Design review of the part built by this model. Coordinates are the model's own, in mm. A direction names the side the tool comes from. Round coordinates to 2 decimals unless told otherwise and drop trailing zeros. Order: outer loops, then holes, each group sorted by start corner. A loop starts at its lowest first (then second) coordinate and runs counter-clockwise, first axis right, second up. Notation, with made-up numbers: (12.25, -4.75) - (20.25, -4.75) arc R30 ccw to (20.25, 33.25) - close; hole circle Ø5 at (21.25, 12). An arc over 180 degrees is marked (long way). Use CSV: the item, a comma, the result in double quotes. Start each with the question number.
from build123d import *

# Parameters (mm, degrees)
F1_DEPTH = 5
F2_R     = 18.5
F3_DEPTH = 9
F4_R     = 16.5
F5_DEPTH = 25
F6_R     = 81
F7_DEPTH = 2.84
F8_R     = 17.4877623158
F9_DEPTH = 25


with BuildPart() as f1:
    # F0 (on Top) → F1 (new body)
    with BuildSketch(Plane.XY):
        with BuildLine():
            Line((18.5, 0), (18.5, 10.68097998))
            Line((18.5, 10.68097998), (9.2500001737, 16.0214698697))
            ThreePointArc((9.2500001737, 16.0214698697), (16.0214700202, 9.2499999131), (18.5, 0))
        make_face()
        with BuildLine():
            ThreePointArc((9.2500002367, -16.0214698334), (16.0214700383, -9.2499998817), (18.5, 0))
            ThreePointArc((18.5, 0), (16.0214700202, 9.2499999131), (9.2500001737, 16.0214698697))
            ThreePointArc((9.2500001737, 16.0214698697), (3.666e-07, 18.5), (-9.2499995387, 16.0214702364))
            ThreePointArc((-9.2499995387, 16.0214702364), (-16.0214698368, 9.2500002307), (-18.5, 0))
            ThreePointArc((-18.5, 0), (-16.0214699908, -9.2499999641), (-9.2500000719, -16.0214699285))
            ThreePointArc((-9.2500000719, -16.0214699285), (9.51e-08, -18.5), (9.2500002367, -16.0214698334))
        make_face()
        with BuildLine():
            Line((18.5, -10.68097998), (18.5, 0))
            ThreePointArc((18.5, 0), (16.0214700383, -9.2499998817), (9.2500002367, -16.0214698334))
            Line((9.2500002367, -16.0214698334), (18.5, -10.68097998))
        make_face()
        with BuildLine():
            ThreePointArc((-9.2499995387, 16.0214702364), (3.666e-07, 18.5), (9.2500001737, 16.0214698697))
            Line((9.2500001737, 16.0214698697), (0, 21.36195996))
            Line((0, 21.36195996), (-9.2499995387, 16.0214702364))
        make_face()
        with BuildLine():
            Line((0, -21.36195996), (9.2500002367, -16.0214698334))
            ThreePointArc((9.2500002367, -16.0214698334), (9.51e-08, -18.5), (-9.2500000719, -16.0214699285))
            Line((-9.2500000719, -16.0214699285), (0, -21.36195996))
        make_face()
        with BuildLine():
            ThreePointArc((-18.5, 0), (-16.0214698368, 9.2500002307), (-9.2499995387, 16.0214702364))
            Line((-9.2499995387, 16.0214702364), (-18.5, 10.68097998))
            Line((-18.5, 10.68097998), (-18.5, 0))
        make_face()
        with BuildLine():
            Line((-18.5, -10.68097998), (-9.2500000719, -16.0214699285))
            ThreePointArc((-9.2500000719, -16.0214699285), (-16.0214699908, -9.2499999641), (-18.5, 0))
            Line((-18.5, 0), (-18.5, -10.68097998))
        make_face()
    extrude(amount=F1_DEPTH)

    # F2 (on face) → F3 (join)
    with BuildSketch(Plane.XY.offset(5)):
        Circle(F2_R)
    extrude(amount=F3_DEPTH)

    # F4 (on face) → F5 (cut)
    with BuildSketch(Plane.XY.offset(14)):
        Circle(F4_R)
    extrude(amount=-F5_DEPTH, mode=Mode.SUBTRACT)

    # F6 (on Top) → F7 (join)
    with BuildSketch(Plane.XY):
        Circle(F6_R)
    extrude(amount=-F7_DEPTH)

    # F8 (on face) → F9 (cut)
    with BuildSketch(Plane.XY):
        Circle(F8_R)
    extrude(amount=-F9_DEPTH, mode=Mode.SUBTRACT)


solid = f1.part
Q1. Tool access review of faces 4 (the flat face through (17, 9, 5)), 5 (the flat face through (18.5, 0, 2)), 6 (the flat face through (17, -10, 5)), 7 (the flat face through (6.4, -15.5, 0)), 8 (the flat face through (-17, -10, 5)): name each direction out of +Z, -Z, +X, -X, +Y, -Y from which nothing blocks a thin tool from reaching the whole face with its end or side.
Q2. Clearance check with flat-ended pins moving along their axes: pin 1 (2 mm diameter, centred on x = 27, y = -49, fed in from +Z); pin 2 (4 mm diameter, centred on y = -2.5, z = 2.5, fed in from +X); pin 3 (5 mm diameter, centred on y = 58.5, z = -1, fed in from +X). State where each tip first meets the part, or that it passes through.
Q3. The part is to be moulded in two halves that separate along X. For faces 1 (the flat face through (-18.5, 0, 2)), 2 (the flat face through (-17, 9, 5)), 3 (the cylindrical face through (15.24, -6.32, 7.1)), say which applies: +X half, -X half, draft (parallel to the pull), parting line (faces both ways), or undercut.
Q4. Take a section at B-B (z = 12). State the section outline as (x, y) points, plus the area to 3 significant figures.
Q5. Take a section at D-D (x = 57.5). State the section outline as (y, z) points, plus the area to 3 significant figures.
Q6. Take a section at C-C (x = -4). State the section outline as (y, z) points.
Q7. Take a section at A-A (y = -5.5). State the section outline as (x, z) points.
Q8. For L1, parallel to Y at x = 0, z = 6.75; L2, parallel to X at y = 1, z = 7.5; L3, parallel to Y at x = 0, z = -1.4, list the stretches that pass through material, from the lowest coordinate up. Write a range as [from, to].
Findings below:
1,face 4,"+Z, +X, +Y"
1,face 5,"+Z, +X, +Y, -Y"
1,face 6,"+Z, +X, -Y"
1,face 7,"-Z"
1,face 8,"+Z, -X, -Y"
2,pin 1,"stops at z = 0"
2,pin 2,"stops at x = 18.5"
2,pin 3,"stops at x = 58.52"
3,face 1,"-X half"
3,face 2,"draft"
3,face 3,"undercut"
4,outline,"circle Ø37 at (0, 0); hole circle Ø33 at (0, 0)"
4,area,"220 mm^2"
5,outline,"(-57.05, -2.84) - (57.05, -2.84) - (57.05, 0) - (-57.05, 0) - close"
5,area,"324 mm^2"
6,outline,"(-80.9, -2.84) - (-17.02, -2.84) - (-17.02, 0) - (-16.01, 0) - (-16.01, 14) - (-18.06, 14) - (-18.06, 5) - (-19.05, 5) - (-19.05, 0) - (-80.9, 0) - close; (16.01, 0) - (17.02, 0) - (17.02, -2.84) - (80.9, -2.84) - (80.9, 0) - (19.05, 0) - (19.05, 5) - (18.06, 5) - (18.06, 14) - (16.01, 14) - close"
7,outline,"(-80.81, -2.84) - (-16.6, -2.84) - (-16.6, 0) - (-15.56, 0) - (-15.56, 14) - (-17.66, 14) - (-17.66, 5) - (-18.5, 5) - (-18.5, 0) - (-80.81, 0) - close; (15.56, 0) - (16.6, 0) - (16.6, -2.84) - (80.81, -2.84) - (80.81, 0) - (18.5, 0) - (18.5, 5) - (17.66, 5) - (17.66, 14) - (15.56, 14) - close"
8,L1,"y = [-18.5, -16.5], [16.5, 18.5]"
8,L2,"x = [-18.47, -16.47], [16.47, 18.47]"
8,L3,"y = [-81, -17.49], [17.49, 81]"
